Model file for the job. Use its own axes, mm. Give positions to 0.01 mm unless a question says otherwise; leave off trailing zeros. Loops run counter-clockwise (first coordinate to the right, second up) from the corner with the lowest first, then second, coordinate; pieces in that order, holes last. Notation, with made-up numbers: (14.25, 86.5) -> (65.25, 86.5) arc R14 cw to (65.25, 98.5) -> close; hole circle Ø8 at (-23, 61). An arc over 180 degrees is marked (long way). Use CSV: the item, a comma, the result in double quotes. Start each with the question number.
(1) Cut at B-B on x = -114. Write the cut outline in (y, z).
(2) Cut at A-A on y = 1.5. State how many separate pieces and enclosed holes the cut face has, then the cut area to 3 significant figures.
(3) Drill centre lines: probe 1 along X at (y, z) = (3.25, -139); probe 2 along Z at (x, y) = (-140, 5); probe 3 along X at (y, z) = (1.75, -206). Where is each one in solid material? Low to high.
(4) Cut at C-C on z = -61. Write the cut outline in (x, y).
(5) Flat gauge pin, fed straight in: pin 1 (3 mm diameter, centred on x = -114, z = -139, fed in from +Y). Where does the tip first touch, or does it go through?
(6) Pull direction X, two halves, no side cores. Call faces 1 (the flat face through (-8, 3, -208)), 2 (the cylindrical face through (-137.52, 3.13, -10.33)), 3 (the flat face through (-138, 3, -207)): pulls with the +X half, pulls with the -X half, needs draft (parallel to the pull), parting line crosses it, or undercut.
from build123d import *

# Parameters (mm, degrees)
SKETCH1_R           = 2.5
BOSS_EXTRUDE1_DEPTH = 6.35


with BuildPart() as part:
    # Sketch1 → Boss-Extrude1 (new body)
    with BuildSketch(Plane(origin=(0, 0, 0), x_dir=(1, 0, 0), z_dir=(0, 1, 0))):
        Polygon((-145, 200), (-130, 215), (-15, 215), (0, 200), (0, 0), (-145, 0), align=None)
        with Locations(Location((-140, 190, 0), (0, 0, 270))):
            Circle(SKETCH1_R, mode=Mode.SUBTRACT)
        with Locations(Location((-114, 190, 0), (0, 0, 270))):
            Circle(SKETCH1_R, mode=Mode.SUBTRACT)
        with Locations(Location((-140, 139, 0), (0, 0, 270))):
            Circle(SKETCH1_R, mode=Mode.SUBTRACT)
        with Locations(Location((-114, 139, 0), (0, 0, 270))):
            Circle(SKETCH1_R, mode=Mode.SUBTRACT)
        with Locations(Location((-31, 190, 0), (0, 0, 270))):
            Circle(SKETCH1_R, mode=Mode.SUBTRACT)
        with Locations(Location((-5, 190, 0), (0, 0, 270))):
            Circle(SKETCH1_R, mode=Mode.SUBTRACT)
        with Locations(Location((-5, 139, 0), (0, 0, 270))):
            Circle(SKETCH1_R, mode=Mode.SUBTRACT)
        with Locations(Location((-31, 139, 0), (0, 0, 270))):
            Circle(SKETCH1_R, mode=Mode.SUBTRACT)
        with Locations(Location((-5, 10, 0), (0, 0, 270))):
            Circle(SKETCH1_R, mode=Mode.SUBTRACT)
        with Locations(Location((-5, 61, 0), (0, 0, 270))):
            Circle(SKETCH1_R, mode=Mode.SUBTRACT)
        with Locations(Location((-31, 61, 0), (0, 0, 270))):
            Circle(SKETCH1_R, mode=Mode.SUBTRACT)
        with Locations(Location((-31, 10, 0), (0, 0, 270))):
            Circle(SKETCH1_R, mode=Mode.SUBTRACT)
        with Locations(Location((-114, 10, 0), (0, 0, 270))):
            Circle(SKETCH1_R, mode=Mode.SUBTRACT)
        with Locations(Location((-114, 61, 0), (0, 0, 270))):
            Circle(SKETCH1_R, mode=Mode.SUBTRACT)
        with Locations(Location((-140, 10, 0), (0, 0, 270))):
            Circle(SKETCH1_R, mode=Mode.SUBTRACT)
        with Locations(Location((-140, 61, 0), (0, 0, 270))):
            Circle(SKETCH1_R, mode=Mode.SUBTRACT)
    extrude(amount=BOSS_EXTRUDE1_DEPTH)


solid = part.part
Check result:
1,outline,"(0, -215) -> (6.35, -215) -> (6.35, -192.5) -> (0, -192.5) -> close; (0, -187.5) -> (6.35, -187.5) -> (6.35, -141.5) -> (0, -141.5) -> close; (0, -136.5) -> (6.35, -136.5) -> (6.35, -63.5) -> (0, -63.5) -> close; (0, -58.5) -> (6.35, -58.5) -> (6.35, -12.5) -> (0, -12.5) -> close; (0, -7.5) -> (6.35, -7.5) -> (6.35, 0) -> (0, 0) -> close"
2,separate pieces,"1"
2,enclosed holes,"16"
2,area,"30,600 mm²"
3,probe 1,"-145 to -142.5, -137.5 to -116.5, -111.5 to -33.5, -28.5 to -7.5, -2.5 to 0"
3,probe 2,"-205 to -192.5, -187.5 to -141.5, -136.5 to -63.5, -58.5 to -12.5, -7.5 to 0"
3,probe 3,"-139 to -6"
4,outline,"(-145, 0) -> (-142.5, 0) -> (-142.5, 6.35) -> (-145, 6.35) -> close; (-137.5, 0) -> (-116.5, 0) -> (-116.5, 6.35) -> (-137.5, 6.35) -> close; (-111.5, 0) -> (-33.5, 0) -> (-33.5, 6.35) -> (-111.5, 6.35) -> close; (-28.5, 0) -> (-7.5, 0) -> (-7.5, 6.35) -> (-28.5, 6.35) -> close; (-2.5, 0) -> (0, 0) -> (0, 6.35) -> (-2.5, 6.35) -> close"
5,pin 1,"through"
6,face 1,"pulls with the +X half"
6,face 2,"undercut"
6,face 3,"pulls with the -X half"
